Can you work these out from the model? Positions are in its coordinate system, mm. A direction names the side the tool comes from. Round coordinates to 2 decimals unless told otherwise and drop trailing zeros. Loops run counter-clockwise (first coordinate to the right, second up) from the corner with the lowest first, then second, coordinate; pieces in that order, holes last. Notation, with made-up numbers: M 51,16 L 97,16 A27 cw 97,35 Z; hole C -38,85.25 d3. An arc over 180 degrees is marked long. Return JSON: item names as keys, results as strings.
```python
from build123d import *

# Parameters (mm, degrees)
BASE_FLANGE1_DEPTH = 100
EDGE_FLANGE1_DEPTH = 197.2
EDGE_FLANGE2_DEPTH = 197.2
HOLE1_START        = -1.4
HOLE1_OUTLINE_R    = 4.5
HOLE1_OUTLINE_R_2  = 1.5
HOLE1_DEPTH        = 102.8
CUT_EXTRUDE2_REACH = 231.743
SKETCH20_R         = 1.21
CUT_EXTRUDE3_REACH = 231.743
SKETCH22_R         = 1.5
SKETCH22_R_2       = 1.87
CUT_EXTRUDE5_REACH = 231.743
SKETCH26_R         = 1.5
CUT_EXTRUDE6_REACH = 231.743
SKETCH27_R         = 1.5
CUT_EXTRUDE7_REACH = 231.743
SKETCH28_R         = 1.5


# Read off the part's stored shape, not the designer's step: Hole1
# Sheet-metal steps are written as plain solids
with BuildPart() as part:
    # Sketch1 → Base-Flange1 (new body)
    with BuildSketch(Plane(origin=(0, 0, 0), x_dir=(1, 0, 0), z_dir=(0, 1, 0))):
        with BuildLine():
            Line((0, 50), (0, 1.4))
            ThreePointArc((0, 1.4), (0.410050506, 0.410050506), (1.4, 0))
            Line((1.4, 0), (198.6, 0))
            ThreePointArc((198.6, 0), (199.589949494, 0.410050506), (200, 1.4))
            Line((200, 1.4), (200, 48.6))
            ThreePointArc((200, 48.6), (199.589949494, 49.589949494), (198.6, 50))
            Line((198.6, 50), (145, 50))
            Line((145, 50), (145, 49.3))
            Line((145, 49.3), (198.6, 49.3))
            ThreePointArc((198.6, 49.3), (199.094974747, 49.094974747), (199.3, 48.6))
            Line((199.3, 48.6), (199.3, 1.4))
            ThreePointArc((199.3, 1.4), (199.094974747, 0.905025253), (198.6, 0.7))
            Line((198.6, 0.7), (1.4, 0.7))
            ThreePointArc((1.4, 0.7), (0.905025253, 0.905025253), (0.7, 1.4))
            Line((0.7, 1.4), (0.7, 50))
            Line((0.7, 50), (0, 50))
        make_face()
    extrude(amount=BASE_FLANGE1_DEPTH)

    # Edge-Flange1 section (across the edge) → Edge-Flange1 (add)
    with BuildSketch(Plane(origin=(198.6, -0.7, -0.7), x_dir=(0, 1, 0), z_dir=(-1, 0, 0))):
        with BuildLine():
            Line((-0.7, 0.7), (-0.7, 49.3))
            Line((-0.7, 49.3), (0, 49.3))
            Line((0, 49.3), (0, 0.7))
            ThreePointArc((0, 0.7), (0.205025253, 0.205025253), (0.7, 0))
            Line((0.7, 0), (0.7, -0.7))
            ThreePointArc((0.7, -0.7), (-0.289949494, -0.289949494), (-0.7, 0.7))
        make_face()
    extrude(amount=EDGE_FLANGE1_DEPTH)

    # Edge-Flange2 section (across the edge) → Edge-Flange2 (add)
    with BuildSketch(Plane(origin=(1.4, 100.7, -0.7), x_dir=(0, -1, 0), z_dir=(1, 0, 0))):
        with BuildLine():
            Line((-0.7, 0.7), (-0.7, 49.3))
            Line((-0.7, 49.3), (0, 49.3))
            Line((0, 49.3), (0, 0.7))
            ThreePointArc((0, 0.7), (0.205025253, 0.205025253), (0.7, 0))
            Line((0.7, 0), (0.7, -0.7))
            ThreePointArc((0.7, -0.7), (-0.289949494, -0.289949494), (-0.7, 0.7))
        make_face()
    extrude(amount=EDGE_FLANGE2_DEPTH)

    # Hole1 outline → Hole1 (cut)
    with BuildSketch(Plane(origin=(0, 0, 0), x_dir=(1, 0, 0), z_dir=(0, 1, 0)).offset(HOLE1_START)):
        with Locations((51.4, 36)):
            Circle(HOLE1_OUTLINE_R)
        with Locations((51.4, 26)):
            Circle(HOLE1_OUTLINE_R_2)
        with Locations((51.4, 46)):
            Circle(HOLE1_OUTLINE_R_2)
    extrude(amount=HOLE1_DEPTH, mode=Mode.SUBTRACT)

    # Sketch20 → Cut-Extrude2 (cut, up to next)
    with BuildSketch(Plane(origin=(0, 0, -50), x_dir=(-1, 0, 0), z_dir=(0, 0, -1)), mode=Mode.PRIVATE) as cut_extrude2_sk1:
        with Locations((-160, 57.75)):
            Circle(SKETCH20_R)
    cut_extrude2_tool1 = extrude(cut_extrude2_sk1.sketch, amount=-CUT_EXTRUDE2_REACH, mode=Mode.PRIVATE) & part.part
    # Sketch20 → Cut-Extrude2 (cut, up to next)
    with BuildSketch(Plane(origin=(0, 0, -50), x_dir=(-1, 0, 0), z_dir=(0, 0, -1)), mode=Mode.PRIVATE) as cut_extrude2_sk2:
        with Locations((-160, 42.25)):
            Circle(SKETCH20_R)
    cut_extrude2_tool2 = extrude(cut_extrude2_sk2.sketch, amount=-CUT_EXTRUDE2_REACH, mode=Mode.PRIVATE) & part.part
    add(cut_extrude2_tool1.solids().sort_by_distance((160, 57.75, -50))[0], mode=Mode.SUBTRACT)
    add(cut_extrude2_tool2.solids().sort_by_distance((160, 42.25, -50))[0], mode=Mode.SUBTRACT)

    # Sketch22 → Cut-Extrude3 (cut, up to next)
    with BuildSketch(Plane.XY, mode=Mode.PRIVATE) as cut_extrude3_sk1:
        with Locations((16.4, 50)):
            Circle(SKETCH22_R)
    cut_extrude3_tool1 = extrude(cut_extrude3_sk1.sketch, amount=-CUT_EXTRUDE3_REACH, mode=Mode.PRIVATE) & part.part
    # Sketch22 → Cut-Extrude3 (cut, up to next)
    with BuildSketch(Plane.XY, mode=Mode.PRIVATE) as cut_extrude3_sk2:
        with Locations((46.4, 50)):
            Circle(SKETCH22_R)
    cut_extrude3_tool2 = extrude(cut_extrude3_sk2.sketch, amount=-CUT_EXTRUDE3_REACH, mode=Mode.PRIVATE) & part.part
    # Sketch22 → Cut-Extrude3 (cut, up to next)
    with BuildSketch(Plane.XY, mode=Mode.PRIVATE) as cut_extrude3_sk3:
        with Locations((66.6, 50)):
            Circle(SKETCH22_R_2)
    cut_extrude3_tool3 = extrude(cut_extrude3_sk3.sketch, amount=-CUT_EXTRUDE3_REACH, mode=Mode.PRIVATE) & part.part
    # Sketch22 → Cut-Extrude3 (cut, up to next)
    with BuildSketch(Plane.XY, mode=Mode.PRIVATE) as cut_extrude3_sk4:
        with Locations((183.6, 50)):
            Circle(SKETCH22_R_2)
    cut_extrude3_tool4 = extrude(cut_extrude3_sk4.sketch, amount=-CUT_EXTRUDE3_REACH, mode=Mode.PRIVATE) & part.part
    add(cut_extrude3_tool1.solids().sort_by_distance((16.4, 50, 0))[0], mode=Mode.SUBTRACT)
    add(cut_extrude3_tool2.solids().sort_by_distance((46.4, 50, 0))[0], mode=Mode.SUBTRACT)
    add(cut_extrude3_tool3.solids().sort_by_distance((66.6, 50, 0))[0], mode=Mode.SUBTRACT)
    add(cut_extrude3_tool4.solids().sort_by_distance((183.6, 50, 0))[0], mode=Mode.SUBTRACT)

    # Sketch26 → Cut-Extrude5 (cut, up to next)
    with BuildSketch(Plane.XY, mode=Mode.PRIVATE) as cut_extrude5_sk1:
        with Locations((5.4, 28.4)):
            Circle(SKETCH26_R)
    cut_extrude5_tool1 = extrude(cut_extrude5_sk1.sketch, amount=-CUT_EXTRUDE5_REACH, mode=Mode.PRIVATE) & part.part
    # Sketch26 → Cut-Extrude5 (cut, up to next)
    with BuildSketch(Plane.XY, mode=Mode.PRIVATE) as cut_extrude5_sk2:
        with Locations((54.9, 28.4)):
            Circle(SKETCH26_R)
    cut_extrude5_tool2 = extrude(cut_extrude5_sk2.sketch, amount=-CUT_EXTRUDE5_REACH, mode=Mode.PRIVATE) & part.part
    # Sketch26 → Cut-Extrude5 (cut, up to next)
    with BuildSketch(Plane.XY, mode=Mode.PRIVATE) as cut_extrude5_sk3:
        with Locations((54.9, 18.4)):
            Circle(SKETCH26_R)
    cut_extrude5_tool3 = extrude(cut_extrude5_sk3.sketch, amount=-CUT_EXTRUDE5_REACH, mode=Mode.PRIVATE) & part.part
    # Sketch26 → Cut-Extrude5 (cut, up to next)
    with BuildSketch(Plane.XY, mode=Mode.PRIVATE) as cut_extrude5_sk4:
        with Locations((5.4, 18.4)):
            Circle(SKETCH26_R)
    cut_extrude5_tool4 = extrude(cut_extrude5_sk4.sketch, amount=-CUT_EXTRUDE5_REACH, mode=Mode.PRIVATE) & part.part
    # Sketch26 → Cut-Extrude5 (cut, up to next)
    with BuildSketch(Plane.XY, mode=Mode.PRIVATE) as cut_extrude5_sk5:
        with Locations((59.4, 23.4)):
            Circle(SKETCH26_R)
    cut_extrude5_tool5 = extrude(cut_extrude5_sk5.sketch, amount=-CUT_EXTRUDE5_REACH, mode=Mode.PRIVATE) & part.part
    add(cut_extrude5_tool1.solids().sort_by_distance((5.4, 28.4, 0))[0], mode=Mode.SUBTRACT)
    add(cut_extrude5_tool2.solids().sort_by_distance((54.9, 28.4, 0))[0], mode=Mode.SUBTRACT)
    add(cut_extrude5_tool3.solids().sort_by_distance((54.9, 18.4, 0))[0], mode=Mode.SUBTRACT)
    add(cut_extrude5_tool4.solids().sort_by_distance((5.4, 18.4, 0))[0], mode=Mode.SUBTRACT)
    add(cut_extrude5_tool5.solids().sort_by_distance((59.4, 23.4, 0))[0], mode=Mode.SUBTRACT)

    # Sketch27 → Cut-Extrude6 (cut, up to next)
    with BuildSketch(Plane.XY, mode=Mode.PRIVATE) as cut_extrude6_sk1:
        with Locations((8.9, 93.7)):
            Circle(SKETCH27_R)
    cut_extrude6_tool1 = extrude(cut_extrude6_sk1.sketch, amount=-CUT_EXTRUDE6_REACH, mode=Mode.PRIVATE) & part.part
    # Sketch27 → Cut-Extrude6 (cut, up to next)
    with BuildSketch(Plane.XY, mode=Mode.PRIVATE) as cut_extrude6_sk2:
        with Locations((8.9, 69.4)):
            Circle(SKETCH27_R)
    cut_extrude6_tool2 = extrude(cut_extrude6_sk2.sketch, amount=-CUT_EXTRUDE6_REACH, mode=Mode.PRIVATE) & part.part
    # Sketch27 → Cut-Extrude6 (cut, up to next)
    with BuildSketch(Plane.XY, mode=Mode.PRIVATE) as cut_extrude6_sk3:
        with Locations((33.9, 93.7)):
            Circle(SKETCH27_R)
    cut_extrude6_tool3 = extrude(cut_extrude6_sk3.sketch, amount=-CUT_EXTRUDE6_REACH, mode=Mode.PRIVATE) & part.part
    # Sketch27 → Cut-Extrude6 (cut, up to next)
    with BuildSketch(Plane.XY, mode=Mode.PRIVATE) as cut_extrude6_sk4:
        with Locations((33.9, 69.4)):
            Circle(SKETCH27_R)
    cut_extrude6_tool4 = extrude(cut_extrude6_sk4.sketch, amount=-CUT_EXTRUDE6_REACH, mode=Mode.PRIVATE) & part.part
    add(cut_extrude6_tool1.solids().sort_by_distance((8.9, 93.7, 0))[0], mode=Mode.SUBTRACT)
    add(cut_extrude6_tool2.solids().sort_by_distance((8.9, 69.4, 0))[0], mode=Mode.SUBTRACT)
    add(cut_extrude6_tool3.solids().sort_by_distance((33.9, 93.7, 0))[0], mode=Mode.SUBTRACT)
    add(cut_extrude6_tool4.solids().sort_by_distance((33.9, 69.4, 0))[0], mode=Mode.SUBTRACT)

    # Sketch28 → Cut-Extrude7 (cut, up to next)
    with BuildSketch(Plane.XY, mode=Mode.PRIVATE) as cut_extrude7_sk1:
        with Locations((194.06, 43.97)):
            Circle(SKETCH28_R)
    cut_extrude7_tool1 = extrude(cut_extrude7_sk1.sketch, amount=-CUT_EXTRUDE7_REACH, mode=Mode.PRIVATE) & part.part
    # Sketch28 → Cut-Extrude7 (cut, up to next)
    with BuildSketch(Plane.XY, mode=Mode.PRIVATE) as cut_extrude7_sk2:
        with Locations((145.8, 45.24)):
            Circle(SKETCH28_R)
    cut_extrude7_tool2 = extrude(cut_extrude7_sk2.sketch, amount=-CUT_EXTRUDE7_REACH, mode=Mode.PRIVATE) & part.part
    # Sketch28 → Cut-Extrude7 (cut, up to next)
    with BuildSketch(Plane.XY, mode=Mode.PRIVATE) as cut_extrude7_sk3:
        with Locations((161.04, 96.04)):
            Circle(SKETCH28_R)
    cut_extrude7_tool3 = extrude(cut_extrude7_sk3.sketch, amount=-CUT_EXTRUDE7_REACH, mode=Mode.PRIVATE) & part.part
    # Sketch28 → Cut-Extrude7 (cut, up to next)
    with BuildSketch(Plane.XY, mode=Mode.PRIVATE) as cut_extrude7_sk4:
        with Locations((188.98, 96.04)):
            Circle(SKETCH28_R)
    cut_extrude7_tool4 = extrude(cut_extrude7_sk4.sketch, amount=-CUT_EXTRUDE7_REACH, mode=Mode.PRIVATE) & part.part
    add(cut_extrude7_tool1.solids().sort_by_distance((194.06, 43.97, 0))[0], mode=Mode.SUBTRACT)
    add(cut_extrude7_tool2.solids().sort_by_distance((145.8, 45.24, 0))[0], mode=Mode.SUBTRACT)
    add(cut_extrude7_tool3.solids().sort_by_distance((161.04, 96.04, 0))[0], mode=Mode.SUBTRACT)
    add(cut_extrude7_tool4.solids().sort_by_distance((188.98, 96.04, 0))[0], mode=Mode.SUBTRACT)


solid = part.part
```
Q1. Thinking about a two-plate mould opening in Y: for faces 6 (the flat face through (101, -1.4, -25)), 7 (the flat face through (99, 101.4, -25)), 8 (the flat face through (101, 49, -0.7)), 9 (the flat face through (199.3, 49, -25)), which applies, pulls with the +Y half, pulls with the -Y half, needs draft (parallel to the pull), parting line crosses it, or undercut?
Results:
{"face 6": "pulls with the -Y half", "face 7": "pulls with the +Y half", "face 8": "undercut", "face 9": "needs draft"}
Q2. On a 3-axis mill with a long thin cutter (end or side, diameter ignored), from which of +Z, -Z, +X, -X, +Y, -Y can I reach the whole of each face in a straight line? I mean faces 1 (the flat face through (171, 49, -49.3)), 2 (the cylindrical face through (50.42, -1.05, -31.61)), 3 (the flat face through (101, -0.7, -26)), 4 (the cylindrical face through (185.327, 49.284, -0.345)), 5 (the flat face through (0.7, 49, -25)). Say none if no direction works.
Results:
{"face 1": "none", "face 2": "+Y, -Y", "face 3": "-Z, +X, -X", "face 4": "+Z", "face 5": "-Z, +Y, -Y"}
Q3. Suppose I cut it at B-B, the plane z = -9. Please give me the cut outline in (x, y), plus the area to 3 significant figures.
Results:
{"outline": "M 0,0 L 0.7,0 L 0.7,100 L 0,100 Z; M 1.4,-1.4 L 198.6,-1.4 L 198.6,-0.7 L 1.4,-0.7 Z; M 1.4,100.7 L 198.6,100.7 L 198.6,101.4 L 1.4,101.4 Z; M 199.3,0 L 200,0 L 200,100 L 199.3,100 Z", "area": "416 mm2"}
Q4. Suppose I cut it at A-A, the plane x = 183.6. Please give me the cut outline in (y, z).
Results:
{"outline": "M -1.4,-50 L -0.7,-50 L -0.7,-1.4 A0.7 cw 0,-0.7 L 48.13,-0.7 L 48.13,0 L 0,0 A1.4 ccw -1.4,-1.4 Z; M 0,-50 L 100,-50 L 100,-49.3 L 0,-49.3 Z; M 51.87,-0.7 L 100,-0.7 A0.7 cw 100.7,-1.4 L 100.7,-50 L 101.4,-50 L 101.4,-1.4 A1.4 ccw 100,0 L 51.87,0 Z"}
Q5. Suppose I cut it at C-C, the plane y = 11.5. Please give me the cut outline in (x, z).
Results:
{"outline": "M 0,-50 L 0.7,-50 L 0.7,-1.4 A0.7 cw 1.4,-0.7 L 198.6,-0.7 A0.7 cw 199.3,-1.4 L 199.3,-48.6 A0.7 cw 198.6,-49.3 L 145,-49.3 L 145,-50 L 198.6,-50 A1.4 ccw 200,-48.6 L 200,-1.4 A1.4 ccw 198.6,0 L 1.4,0 A1.4 ccw 0,-1.4 Z"}
Q6. If I drill on line 1 along Z through (x, y) = (170, 14); line 2 along Y through (x, z) = (149, -35.5); line 3 along X through (y, z) = (39, -3.5), over which ranges is the centre line in solid material (lowest first)?
Results:
{"line 1": "z = -50 to -49.3, -0.7 to 0", "line 2": "y = -1.4 to -0.7, 100.7 to 101.4", "line 3": "x = 0 to 0.7, 199.3 to 200"}
Q7. Suppose I cut it at D-D, the plane z = -36. Please give me the cut outline in (x, y), plus the area to 3 significant figures.
Results:
{"outline": "M 0,0 L 0.7,0 L 0.7,100 L 0,100 Z; M 1.4,-1.4 L 46.9,-1.4 L 46.9,-0.7 L 1.4,-0.7 Z; M 1.4,100.7 L 46.9,100.7 L 46.9,101.4 L 1.4,101.4 Z; M 55.9,-1.4 L 198.6,-1.4 L 198.6,-0.7 L 55.9,-0.7 Z; M 55.9,100.7 L 198.6,100.7 L 198.6,101.4 L 55.9,101.4 Z; M 199.3,0 L 200,0 L 200,100 L 199.3,100 Z", "area": "403 mm2"}
Q8. I'm going to push flat-ended pins straight in: pin 1 Ø6 at (x, y) = (66.6, 50) entering from -Z; pin 2 Ø2 at (x, y) = (183.6, 50) entering from +Z; pin 3 Ø1.5 at (y, z) = (101, -29.5) entering from +X. Where does each tip first touch, or does it pass through?
Results:
{"pin 1": "stops at z = -0.7", "pin 2": "stops at z = -49.3", "pin 3": "stops at x = 198.6"}
